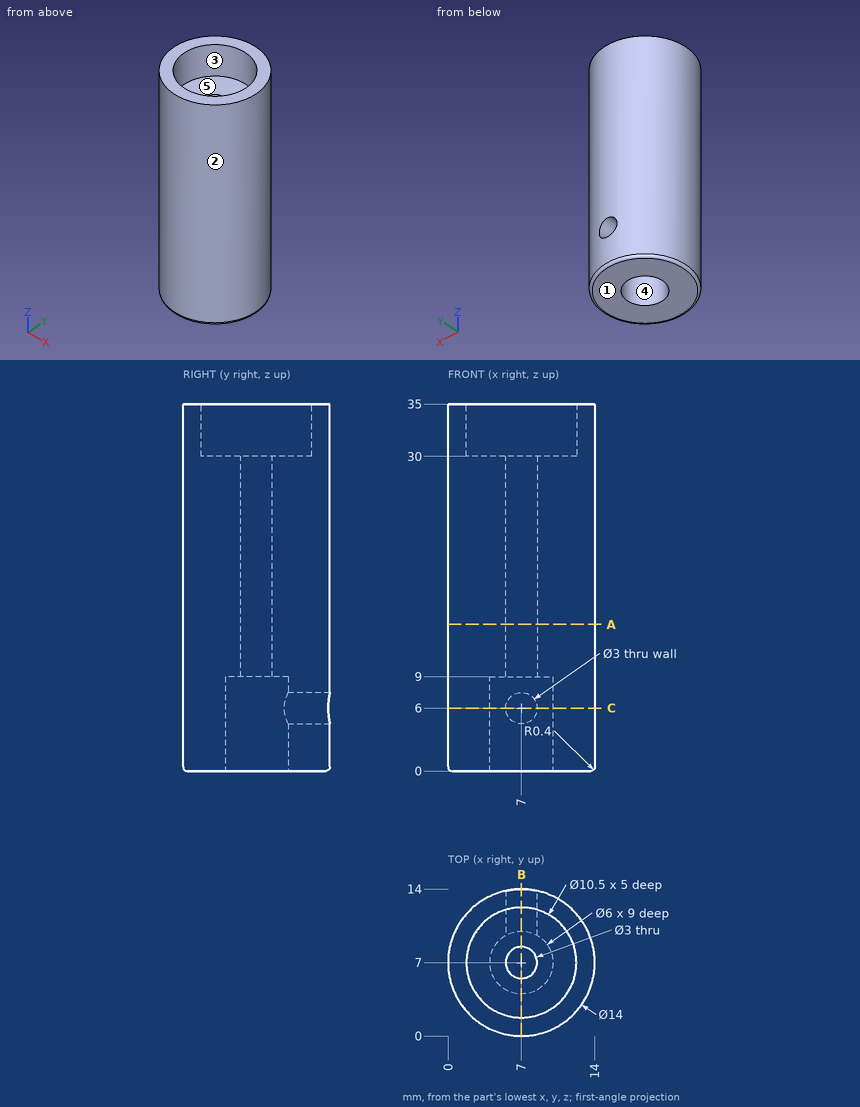
Design review of the part shown in the three views and the two pictorial views. Dimensions are in mm from the part's minimum x, y and z. A direction names the side the tool comes from. Round coordinates to 2 decimals unless told otherwise and drop trailing zeros. Loops run counter-clockwise (first coordinate to the right, second up) from the corner with the lowest first, then second, coordinate; pieces in that order, holes last.
(1) We need section C-C (z = 6). Give the boundary of the cut face in (x, y), plus the area to 3 significant figures.
Returned:
outline: (5.5, 9.6) - (5.5, 13.84) arc R7 ccw (long way) to (8.5, 13.84) - (8.5, 9.6) arc R3 cw (long way) to start
area: 113 mm2
(2) We need section B-B (x = 7). State how many separate pieces and enclosed holes the cut face has, plus the area to 3 significant figures.
Returned:
separate pieces: 3
enclosed holes: 0
area: 308 mm2
(3) Tool access review of the marked faces 4 and 5: name each direction out of +Z, -Z, +X, -X, +Y, -Y from which nothing blocks a thin tool from reaching the whole face with its end or side.
Returned:
face 4: -Z
face 5: +Z
(4) Clearance check with flat-ended pins moving along their axes: P1, Ø1, axis at y = 3, z = 30, coming from the -X side; P2, Ø2, axis at y = 4.5, z = 23.5, coming from the +X side; P3, Ø3, axis at x = 7.5, y = 7, coming from the -Z side. State where each tip first meets the part, or that it passes through.
Returned:
P1: stops at x = 0.94
P2: stops at x = 13.84
P3: stops at z = 9
(5) We need section A-A (z = 14). Give the boundary of the cut face in (x, y), plus the area to 3 significant figures.
Returned:
outline: circle Ø14 at (7, 7); hole circle Ø3 at (7, 7)
area: 147 mm2
(6) Mouldability with a two-part tool opening along Y and no side actions: class the marked faces 1, 2 and 3 as released by +Y, released by -Y, zero draft, split by the parting line, or undercut.
Returned:
face 1: zero draft
face 2: split by the parting line
face 3: undercut
(7) Wall thickness on line 1 along Y through (x, z) = (7, 33.6); line 2 along Y through (x, z) = (7, 5.5); line 3 along Z through (x, y) = (7, 9): over which ranges is each line inside the solid? List them lowest first.
Returned:
line 1: y = 0 to 1.75, 12.25 to 14
line 2: y = 0 to 4
line 3: z = 9 to 30
